```python
from build123d import *

# Parameters (mm, degrees)
SKETCH1_R           = 6.6675
BOSS_EXTRUDE1_DEPTH = 1.905
BOSS_EXTRUDE2_DEPTH = 3.175
SKETCH3_R           = 6.35
CUT_EXTRUDE1_DEPTH  = 14.145931484
FILLET1_R           = 1.27
FILLET2_R           = 0.381
FILLET3_R           = 0.381
FILLET4_R           = 0.127
FILLET5_R           = 0.127


with BuildPart() as part:
    # Sketch1 → Boss-Extrude1 (new body)
    with BuildSketch(Plane.XY):
        with Locations(Location((0, 0, 0), (0, 0, 180))):
            Circle(SKETCH1_R)
    extrude(amount=BOSS_EXTRUDE1_DEPTH)

    # Sketch2 → Boss-Extrude2 (add)
    with BuildSketch(Plane.XY.offset(1.905)):
        Polygon((0, -9.165435523), (7.9375, -4.582717762), (7.9375, 4.582717762), (0, 9.165435523), (-7.9375, 4.582717762), (-7.9375, -4.582717762), align=None)
    extrude(amount=BOSS_EXTRUDE2_DEPTH)

    # Sketch3 → Cut-Extrude1 (cut, through all)
    with BuildSketch(Plane(origin=(0, 0, 0), x_dir=(-1, 0, 0), z_dir=(0, 0, -1))):
        Circle(SKETCH3_R)
    extrude(amount=-CUT_EXTRUDE1_DEPTH, mode=Mode.SUBTRACT)

    # Fillet1
    fillet1_edges = [part.edges().sort_by_distance(p)[0] for p in [
        (-7.9375, -4.582717762, 3.4925),
        (0, -9.165435523, 3.4925),
        (7.9375, -4.582717762, 3.4925),
        (7.9375, 4.582717762, 3.4925),
        (0, 9.165435523, 3.4925),
        (-7.9375, 4.582717762, 3.4925),
    ]]
    fillet(fillet1_edges, radius=FILLET1_R)

    # Fillet2
    fillet2_edges = [part.edges().sort_by_distance(p)[0] for p in [
        (-7.9375, 0, 1.905),
        (-3.96875, -6.874076643, 1.905),
        (-3.96875, 6.874076643, 1.905),
        (3.96875, 6.874076643, 1.905),
        (7.9375, 0, 1.905),
        (3.96875, -6.874076643, 1.905),
        (0, 8.96896584, 1.905),
        (7.767352263, 4.48448292, 1.905),
        (7.767352263, -4.48448292, 1.905),
        (0, -8.96896584, 1.905),
        (-7.767352263, -4.48448292, 1.905),
        (-7.767352263, 4.48448292, 1.905),
    ]]
    fillet(fillet2_edges, radius=FILLET2_R)

    # Fillet3
    fillet3_edges = [part.edges().sort_by_distance(p)[0] for p in [
        (-7.9375, 0, 5.08),
        (-3.96875, 6.874076643, 5.08),
        (-3.96875, -6.874076643, 5.08),
        (3.96875, -6.874076643, 5.08),
        (7.9375, 0, 5.08),
        (3.96875, 6.874076643, 5.08),
        (0, 8.96896584, 5.08),
        (7.767352263, 4.48448292, 5.08),
        (7.767352263, -4.48448292, 5.08),
        (0, -8.96896584, 5.08),
        (-7.767352263, -4.48448292, 5.08),
        (-7.767352263, 4.48448292, 5.08),
    ]]
    fillet(fillet3_edges, radius=FILLET3_R)

    # Fillet4
    fillet4_edges = [part.edges().sort_by_distance(p)[0] for p in [
        (6.35, 0, 5.08),
    ]]
    fillet(fillet4_edges, radius=FILLET4_R)

    # Fillet5
    fillet5_edges = [part.edges().sort_by_distance(p)[0] for p in [
        (6.6675, 0, 0),
        (6.6675, 0, 1.905),
    ]]
    fillet(fillet5_edges, radius=FILLET5_R)


solid = part.part
```
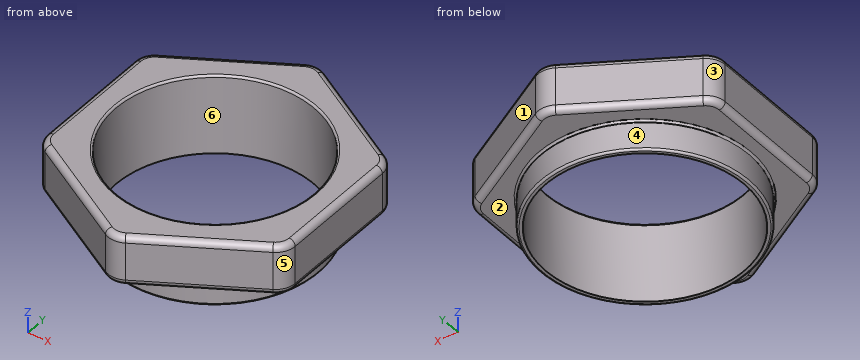
Source: CAD feature listing. Evaluate the final solid. Frame: model axes, mm. Face numbers are marked on the shaded views. A direction names the side the tool comes from. Coordinates: 2 decimals unless noted, no trailing zeros. Use a Markdown table: item, result. Add a question column.
Q1. Material intervals for L1, parallel to Y at x = 0, z = 2.95; L2, parallel to Y at x = 0, z = 1.4; L3, parallel to Z at x = -3.5, y = -6.25 (3 decimals), sorted ascending.
Q2. First-contact query: pin 1 (1.5 mm diameter, centred on y = 6.5, z = 1.5, fed in from -X); pin 2 (2 mm diameter, centred on x = 4, z = 2.5, fed in from +Y); pin 3 (1.5 mm diameter, centred on x = -4, z = 2.5, fed in from -Y). Flat tips, straight axial feed; report the tip coordinate or a pass-through.
Q3. Access query for the marked faces 1 and 2. Directions: +Z, -Z, +X, -X, +Y, -Y. A direction counts if a zero-diameter tool reaches every point of the face in a straight line with its end or side. Return the directions, or none.
Q4. Draft query along Y for the marked faces 3, 4, 5 and 6. Return one class per face: pulls with the +Y half, pulls with the -Y half, needs draft (parallel to the pull), parting line crosses it, or undercut.
Result:
| question | item | result |
|---|---|---|
| 1 | L1 | y = -8.97 to -6.35, 6.35 to 8.97 |
| 1 | L2 | y = -6.67 to -6.35, 6.35 to 6.67 |
| 1 | L3 | z = 1.905 to 5.08 |
| 2 | pin 1 | stops at x = -5.34 |
| 2 | pin 2 | stops at y = 7.43 |
| 2 | pin 3 | stops at y = -7.29 |
| 3 | face 1 | +Z, -Z, +X, +Y |
| 3 | face 2 | -Z |
| 4 | face 3 | pulls with the +Y half |
| 4 | face 4 | parting line crosses it |
| 4 | face 5 | pulls with the -Y half |
| 4 | face 6 | undercut |
